Read the model definition and answer for the solid it produces. Units are mm, in the model's axes. A direction names the side the tool comes from. Give positions to 0.01 mm unless a question says otherwise; leave off trailing zeros. Order: outer loops, then holes, each group sorted by start corner. A loop starts at its lowest first (then second) coordinate and runs counter-clockwise, first axis right, second up.
```python
from build123d import *

# Parameters (mm, degrees)
ESQUISSE1_RX            = 42.396864719
ESQUISSE1_RY            = 41.029112223
ESQUISSE1_RX_2          = 31.648634461
ESQUISSE1_RY_2          = 29.877092437
BOSS_EXTRU_1_DEPTH      = 170
ESQUISSE2_W             = 15.792738377
ESQUISSE2_H             = 16.344932025
ESQUISSE2_W_2           = 18.553706624
ESQUISSE2_H_2           = 11.816944099
ENL_V_MAT_EXTRU_1_DEPTH = 170
ESQUISSE3_R             = 11.193216681
BOSS_EXTRU_2_DEPTH      = 170


with BuildPart() as part:
    # Esquisse1 → Boss.-Extru.1 (new body)
    with BuildSketch(Plane.XY):
        with Locations(Location((0, 0), (0, 0, 37.303948278))):
            Ellipse(ESQUISSE1_RX, ESQUISSE1_RY)
        with Locations(Location((0, 0), (0, 0, -25.781336929))):
            Ellipse(ESQUISSE1_RX_2, ESQUISSE1_RY_2, mode=Mode.SUBTRACT)
    extrude(amount=BOSS_EXTRU_1_DEPTH)

    # Esquisse2 → Enlèv. mat.-Extru.1 (cut)
    with BuildSketch(Plane.XY.offset(170)):
        with Locations((2.926626343, 29.21104406)):
            Rectangle(ESQUISSE2_W, ESQUISSE2_H)
        with Locations((-0.22087746, -41.635401174)):
            Rectangle(ESQUISSE2_W_2, ESQUISSE2_H_2)
    extrude(amount=-ENL_V_MAT_EXTRU_1_DEPTH, mode=Mode.SUBTRACT)

    # Esquisse3 → Boss.-Extru.2 (add)
    with BuildSketch(Plane.XY.offset(170)):
        with Locations((-46.482294325, 0)):
            Circle(ESQUISSE3_R)
    extrude(amount=-BOSS_EXTRU_2_DEPTH)


solid = part.part
```
1) The part is cut by section A-A on x = -49. Determine the outline of the cut face in (y, z).
Final values:
outline: (-10.91, 0) - (10.91, 0) - (10.91, 170) - (-10.91, 170) - close
2) Consider L1, parallel to Y at x = 0, z = 142; L2, parallel to X at y = -2, z = 22.5; L3, parallel to X at y = -22.5, z = 132. Determine where each line is inside the solid, lowest interval first.
Final values:
L1: y = -35.73 to -30.19, 37.38 to 41.52
L2: x = -57.5 to -31.13, 31.31 to 41.77
L3: x = -35.92 to -19.84, 21.94 to 34.49
3) Given pin 1 (8 mm diameter, centred on y = 35, z = 48, fed in from +X); pin 2 (2.5 mm diameter, centred on y = -38.5, z = 99, fed in from -X); pin 3 (2 mm diameter, centred on x = 28.5, y = -0.5, fed in from -Z); pin 4 (10 mm diameter, centred on x = 20, z = 102, fed in from -Y), each flat-ended and moving along its own axis, determine where each tip first touches the part or whether it passes through.
Final values:
pin 1: stops at x = 28.86
pin 2: stops at x = -19.72
pin 3: passes through
pin 4: stops at y = -38.29
4) A tool of negligible diameter and unlimited length cuts with its end or side. For faces 4 (the face through (-31, -8, 170)), 5 (the face through (-4.97, 34, 86)), 6 (the face through (-9.498, -38, 86)), from which of +Z, -Z, +X, -X, +Y, -Y can it reach the whole face along a straight path? Write none if from no direction.
Final values:
face 4: +Z, +X, -X, +Y, -Y
face 5: +Z, -Z
face 6: +Z, -Z, -Y
5) For a pull along Y with two mould halves and no side action, classify faces 1 (the face through (9.056, -38, 86)), 2 (the face through (0, -35.727, 86)), 3 (the face through (10.823, 33, 86)) as released by +Y, released by -Y, zero draft, split by the parting line, or undercut.
Final values:
face 1: zero draft
face 2: released by -Y
face 3: undercut
